from build123d import *

# Parameters (mm, degrees)
BOSS_EXTRUDE1_DEPTH = 6


with BuildPart() as part:
    # Sketch1 → Boss-Extrude1 (new body)
    with BuildSketch(Plane(origin=(0, 0, 0), x_dir=(1, 0, 0), z_dir=(0, 1, 0))):
        with BuildLine():
            Line((0, -55), (225, -55))
            ThreePointArc((225, -55), (263.890872965, -38.890872965), (280, 0))
            Line((280, 0), (280, 90))
            ThreePointArc((280, 90), (263.890872965, 128.890872965), (225, 145))
            Line((225, 145), (0, 145))
            ThreePointArc((0, 145), (-38.890872965, 128.890872965), (-55, 90))
            Line((-55, 90), (-55, 0))
            ThreePointArc((-55, 0), (-38.890872965, -38.890872965), (0, -55))
        make_face()
        with BuildLine():
            Line((0, -30), (225, -30))
            ThreePointArc((225, -30), (246.213203436, -21.213203436), (255, 0))
            Line((255, 0), (255, 60))
            Line((255, 60), (165, 60))
            Line((165, 60), (165, 90))
            ThreePointArc((165, 90), (156.213203436, 111.213203436), (135, 120))
            Line((135, 120), (0, 120))
            ThreePointArc((0, 120), (-21.213203436, 111.213203436), (-30, 90))
            Line((-30, 90), (-30, 0))
            ThreePointArc((-30, 0), (-21.213203436, -21.213203436), (0, -30))
        make_face(mode=Mode.SUBTRACT)
    extrude(amount=BOSS_EXTRUDE1_DEPTH)


solid = part.part
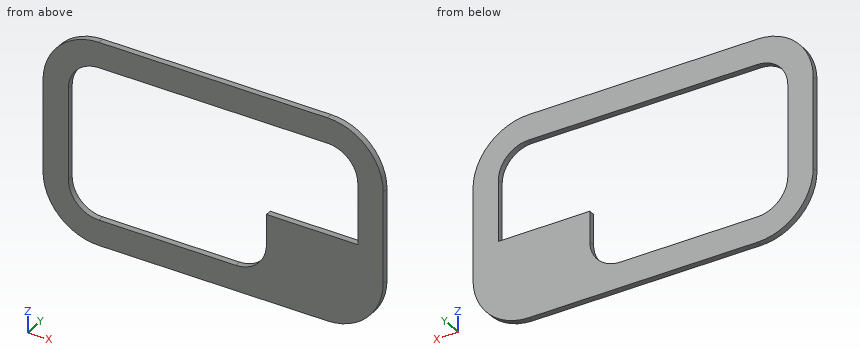
Source: CAD feature listing. Evaluate the final solid. Frame: model axes, mm. Coordinates: 2 decimals unless noted, no trailing zeros. Order: outer loops, then holes, each group sorted by start corner. A loop starts at its lowest first (then second) coordinate and runs counter-clockwise, first axis right, second up.
Item 1: Cut plane A-A (z = -38). Return loops of the section in (x, y).
Output values:
outline: (-55, 0) - (-30, 0) - (-30, 6) - (-55, 6) - close; (255, 0) - (280, 0) - (280, 6) - (255, 6) - close
Item 2: First-contact query: P1, Ø3, axis at x = -10.5, y = 4.5, coming from the -Z side. Flat tip, straight axial feed; report the tip coordinate or a pass-through.
Output values:
P1: stops at z = -144.26
Item 3: Material intervals for line 1 (X direction, y = 4.8, z = -4); line 2 (X direction, y = 1.75, z = -67); line 3 (Z direction, x = 44, y = 0.65), sorted ascending.
Output values:
line 1: x = -55 to -30, 255 to 280
line 2: x = -55 to -30, 165 to 280
line 3: z = -145 to -120, 30 to 55
Item 4: Cut plane B-B (x = 131). Return loops of the section in (y, z), plus the area to 3 significant figures.
Output values:
outline: (0, -145) - (6, -145) - (6, -120) - (0, -120) - close; (0, 30) - (6, 30) - (6, 55) - (0, 55) - close
area: 300 mm2
Item 5: Cut plane C-C (y = 2.2). Return loops of the section in (x, z).
Output values:
outline: (-55, -90) arc R55 ccw to (0, -145) - (225, -145) arc R55 ccw to (280, -90) - (280, 0) arc R55 ccw to (225, 55) - (0, 55) arc R55 ccw to (-55, 0) - close; hole (-30, -90) arc R30 ccw to (0, -120) - (135, -120) arc R30 ccw to (165, -90) - (165, -60) - (255, -60) - (255, 0) arc R30 ccw to (225, 30) - (0, 30) arc R30 ccw to (-30, 0) - close
Item 6: Cut plane D-D (z = 36). Return loops of the section in (x, y), plus the area to 3 significant figures.
Output values:
outline: (-41.58, 0) - (266.58, 0) - (266.58, 6) - (-41.58, 6) - close
area: 1,850 mm2
